For this review, take the finished solid that the model builds, in its own axes (mm). Face numbers are marked on the shaded views. A direction names the side the tool comes from. Give positions to 0.01 mm unless a question says otherwise; leave off trailing zeros. Write each loop counter-clockwise with the first axis right and the second up, starting at its lowest first coordinate (ties: lowest second). Pieces come first, ordered by that corner, then holes.
Q1. Insertion check: P1, Ø3.5, axis at x = -21.5, z = 28.5, coming from the -Y side; P2, Ø6, axis at y = -54.5, z = 14, coming from the -X side; P3, Ø2, axis at y = -6.5, z = -4, coming from the +X side; P4, Ø6.5, axis at y = -50.5, z = 30.5, coming from the -X side. Each pin has a flat end and moves straight along its axis. Give the tip position at first contact, or say it passes through.
Q2. We need section A-A (y = -12.5). Give the number of separate pieces and of enclosed holes in the cut face, then the cut area to 3 significant figures.
Q3. For line 1 (X direction, y = -34.5, z = 25.5); line 2 (X direction, y = -20, z = 0) (3 decimals); line 3 (Y direction, x = 6, z = -21) (3 decimals), list the stretches that pass through material, from the lowest coordinate up.
Q4. Mouldability with a two-part tool opening along Y and no side actions: class the marked faces 5, 6 and 7 as released by +Y, released by -Y, zero draft, split by the parting line, or undercut.
Q5. We need section C-C (y = -2). Write out the cut boundary in (x, z), then the cut area to 3 significant figures.
Q6. Machinability: for the marked faces 1, 2, 3 and 4, which of the approach directions +Z, -Z, +X, -X, +Y, -Y give a long, thin tool a straight path to every point of the face, cutting with its end or side? Answer none if there is none.
```python
from build123d import *

# Parameters (mm, degrees)
BASE_EXTRUDE_DEPTH              = 33.02
SKETCH3_OUTSIDE_W               = 90.796
SKETCH3_OUTSIDE_H               = 92.225
CUT_EXTRUDE1_DEPTH              = 84.020179032
FILLET1_R                       = 3.175
SHELL1_START                    = -64
SHELL1_DEPTH                    = 60.825
CUT_EXTRUDE2_DEPTH              = 90.002703004
BOSS_EXTRUDE2_REACH             = 82.294
SKETCH5_R                       = 4.7625
BOSS_EXTRUDE2_DIRECTION_2_REACH = 82.294
BOSS_EXTRUDE3_DEPTH             = 3.175
SKETCH7_R                       = 6.35
BOSS_EXTRUDE4_DEPTH             = 4.7625


with BuildPart() as part:
    # Sketch2 → Base-Extrude (new, symmetric)
    with BuildSketch(Plane.ZY):
        with BuildLine():
            Line((-25.4, 0), (31.75, 0))
            Line((31.75, 0), (41.801384237, -48.20777973))
            ThreePointArc((41.801384237, -48.20777973), (33.708556891, -62.735496477), (18.174681196, -56.798568464))
            ThreePointArc((18.174681196, -56.798568464), (-0.820496403, -29.162568375), (-25.4, -6.35))
            Line((-25.4, -6.35), (-25.4, 0))
        make_face()
    extrude(amount=BASE_EXTRUDE_DEPTH, both=True)

    # Sketch3 outside → Cut-Extrude1 (cut, through all)
    with BuildSketch(Plane(origin=(0, 0, 0), x_dir=(-1, 0, 0), z_dir=(0, 1, 0))):
        with Locations((0, 8.3345)):
            Rectangle(SKETCH3_OUTSIDE_W, SKETCH3_OUTSIDE_H)
        with BuildLine():
            Line((20.6375, 14.807214247), (20.6375, 48.151384237))
            Line((20.6375, 48.151384237), (-20.6375, 48.151384237))
            Line((-20.6375, 48.151384237), (-20.6375, 14.807214247))
            ThreePointArc((-20.6375, 14.807214247), (0, -25.4), (20.6375, 14.807214247))
        make_face(mode=Mode.SUBTRACT)
    extrude(amount=-CUT_EXTRUDE1_DEPTH, mode=Mode.SUBTRACT)

    # Fillet1
    # the kernel refuses this fillet: 3.175 mm, written as the material it adds along each edge
    with BuildSketch(Plane(origin=(20.6375, 0, 14.807214247), x_dir=(0.567961525786319, 0, -0.8230551046111534), z_dir=(0, -1, 0))) as fillet1_piece_1_section:
        with BuildLine():
            CenterArc((0.989925475, 3.174465965), FILLET1_R, 235.391801271, 33.557309762)
            Line((-0.813352369, 0.561266008), (0, 0))
            ThreePointArc((0, 0), (0.465847282, 0.004272282), (0.931694565, 0))
        make_face()
    fillet1_piece_1 = extrude(amount=53.310385567, mode=Mode.PRIVATE)
    fillet1_piece_1 = fillet1_piece_1 - Plane(origin=(20.6375, -128.781390034, -116.154144448), x_dir=(0, 0.4723282255219985, 0.8814227404459453), z_dir=(-1, 0, 0)) * Cylinder(152.4, 111, mode=Mode.PRIVATE)
    add(fillet1_piece_1)
    with BuildSketch(Plane(origin=(-20.6375, 0, 14.807214247), x_dir=(-0.5679615257863165, 0, -0.8230551046111549), z_dir=(0, -1, 0))) as fillet1_piece_2_section:
        with BuildLine():
            CenterArc((0.989925475, -3.174465965), FILLET1_R, 91.050888967, 33.557309762)
            Line((-0.813352369, -0.561266008), (0, 0))
            ThreePointArc((0, 0), (0.465847282, -0.004272282), (0.931694565, 0))
        make_face()
    fillet1_piece_2 = extrude(amount=53.310385567, mode=Mode.PRIVATE)
    fillet1_piece_2 = fillet1_piece_2 - Plane(origin=(-20.6375, -128.781390034, -116.154144448), x_dir=(0, 0.4723282255219985, 0.8814227404459453), z_dir=(-1, 0, 0)) * Cylinder(152.4, 111, mode=Mode.PRIVATE)
    add(fillet1_piece_2)
    # the kernel refuses this fillet: 3.175 mm, written as the material it takes off along each edge
    with BuildSketch(Plane(origin=(0, 0, 0), x_dir=(-0.8333333333333335, 0, 0.5527707983925666), z_dir=(0.5527707983925666, 0, 0.8333333333333335))) as fillet1_2_piece_1:
        with BuildLine():
            CenterArc((25.4 - FILLET1_R, FILLET1_R), FILLET1_R, 270, 90)
            Line((25.4 - FILLET1_R, 0), (25.4, 0))
            Line((25.4, 0), (25.4, FILLET1_R))
        make_face()
    revolve(axis=Axis((0, 0, 0), (0, -1, 0)), revolution_arc=247.114619524, mode=Mode.SUBTRACT)
    with BuildSketch(Plane(origin=(20.6375, 0, 39.6875), x_dir=(-1, 0, 0), z_dir=(0, 0, -1)), Plane(origin=(-20.6375, 0, 15.795425564), x_dir=(1, 0, 0), z_dir=(0, 0, 1))) as fillet1_2_piece_2:
        with BuildLine():
            CenterArc((FILLET1_R, -FILLET1_R), FILLET1_R, 90, 90)
            Line((0, -FILLET1_R), (0, 0))
            Line((0, 0), (FILLET1_R, 0))
        make_face()
    extrude(amount=23.892074436, mode=Mode.SUBTRACT)
    with BuildSketch(Plane(origin=(-23.8125, 0, 15.795425564), x_dir=(0.8333333333333333, 0, -0.5527707983925668), z_dir=(-0.5527707983925668, 0, -0.8333333333333333))) as fillet1_2_piece_3:
        with BuildLine():
            CenterArc((3.175 + FILLET1_R, FILLET1_R), FILLET1_R, 180, 90)
            Line((3.175, FILLET1_R), (3.175, 0))
            Line((3.175, 0), (3.175 + FILLET1_R, 0))
        make_face()
    revolve(axis=Axis((-23.8125, 0, 15.795425564), (0, -1, 0)), revolution_arc=33.557309762, mode=Mode.SUBTRACT)
    with BuildSketch(Plane(origin=(23.8125, 0, 15.795425564), x_dir=(-0.8333333333333333, 0, -0.5527707983925668), z_dir=(0.5527707983925668, 0, -0.8333333333333333))) as fillet1_2_piece_4:
        with BuildLine():
            CenterArc((3.175 + FILLET1_R, -FILLET1_R), FILLET1_R, 90, 90)
            Line((3.175, -FILLET1_R), (3.175, 0))
            Line((3.175, 0), (3.175 + FILLET1_R, 0))
        make_face()
    revolve(axis=Axis((23.8125, 0, 15.795425564), (0, 1, 0)), revolution_arc=33.557309762, mode=Mode.SUBTRACT)

    # Shell1: read off the stored shape, not the designer's step
    # Shell1 outline → Shell1 (cut)
    with BuildSketch(Plane(origin=(0, 0, 0), x_dir=(1, 0, 0), z_dir=(0, 1, 0)).offset(SHELL1_START)):
        with BuildLine():
            ThreePointArc((17.4625, -15.795425564), (17.732837866, -13.962338459), (18.520833333, -12.285330994))
            ThreePointArc((18.520833333, -12.285330994), (0, 22.225), (-18.520833333, -12.285330994))
            ThreePointArc((-18.520833333, -12.285330994), (-17.732837866, -13.962338459), (-17.4625, -15.795425564))
            Line((-17.4625, -15.795425564), (-17.4625, -44))
            Line((-17.4625, -44), (17.4625, -44))
            Line((17.4625, -44), (17.4625, -15.795425564))
        make_face()
    extrude(amount=SHELL1_DEPTH, mode=Mode.SUBTRACT)

    # Sketch4 → Cut-Extrude2 (cut, through all)
    with BuildSketch(Plane.ZY.offset(-20.6375)):
        with BuildLine():
            Line((24.14125847, -10.173055068), (28.029588875, -28.822006423))
            ThreePointArc((28.029588875, -28.822006423), (31.785802502, -31.282109915), (34.245905994, -27.525896288))
            Line((34.245905994, -27.525896288), (30.357575589, -8.876944932))
            ThreePointArc((30.357575589, -8.876944932), (26.601361962, -6.416841441), (24.14125847, -10.173055068))
        make_face()
    extrude(amount=CUT_EXTRUDE2_DEPTH, mode=Mode.SUBTRACT)

    # Sketch5 → Boss-Extrude2 (add, up to next)
    with BuildSketch(Plane(origin=(0, 0, 0), x_dir=(0, 0, -1), z_dir=(1, 0, 0)), mode=Mode.PRIVATE) as boss_extrude2_sk1:
        with Locations((-29.36875, -50.8)):
            Circle(SKETCH5_R)
    boss_extrude2_tool1 = extrude(boss_extrude2_sk1.sketch, amount=BOSS_EXTRUDE2_REACH, mode=Mode.PRIVATE) - part.part
    add(boss_extrude2_tool1.solids().sort_by_distance((0, -50.8, 29.36875))[0])

    # Sketch5 → Boss-Extrude2 direction 2 (add, up to next)
    with BuildSketch(Plane(origin=(0, 0, 0), x_dir=(0, 0, -1), z_dir=(1, 0, 0)), mode=Mode.PRIVATE) as boss_extrude2_direction_2_sk1:
        with Locations((-29.36875, -50.8)):
            Circle(SKETCH5_R)
    boss_extrude2_direction_2_tool1 = extrude(boss_extrude2_direction_2_sk1.sketch, amount=-BOSS_EXTRUDE2_DIRECTION_2_REACH, mode=Mode.PRIVATE) - part.part
    add(boss_extrude2_direction_2_tool1.solids().sort_by_distance((0, -50.8, 29.36875))[0])

    # Sketch6 → Boss-Extrude3 (add)
    with BuildSketch(Plane.ZY.offset(20.6375)):
        Polygon((33.034924209, -44.45), (25.702575791, -44.45), (22.036401581, -50.8), (25.702575791, -57.15), (33.034924209, -57.15), (36.701098419, -50.8), align=None)
    boss_extrude3 = extrude(amount=BOSS_EXTRUDE3_DEPTH)

    # Mirror1: Boss-Extrude3 across plane
    add(boss_extrude3.mirror(Plane(origin=(0, 0, 0), x_dir=(0, 0, 1), z_dir=(1, 0, 0))))

    # Sketch7 → Boss-Extrude4 (add)
    with BuildSketch(Plane(origin=(0, 0, 0), x_dir=(-1, 0, 0), z_dir=(0, 1, 0))):
        with Locations(Location((0, 0, 0), (0, 0, 270))):
            Circle(SKETCH7_R)
    extrude(amount=BOSS_EXTRUDE4_DEPTH)


solid = part.part
```
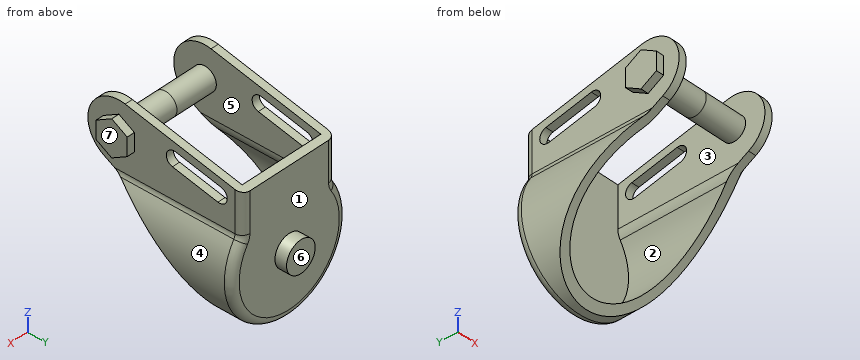
Computed:
1. P1: stops at y = -63.5
1. P2: stops at x = -20.66
1. P3: stops at x = 25.22
1. P4: stops at x = -23.81
2. separate pieces: 4
2. enclosed holes: 0
2. area: 309 mm2
3. line 1: x = -20.64 to -17.46, 17.46 to 20.64
3. line 2: x = -25.4 to -22.225, 22.225 to 25.4
3. line 3: y = -3.175 to 0
4. face 5: undercut
4. face 6: released by +Y
4. face 7: zero draft
5. outline: (-20.98, 13.92) arc R25.17 ccw (long way) to (20.98, 13.92) arc R3.4 cw to (20.41, 15.8) - (20.41, 32.17) - (-20.41, 32.17) - (-20.41, 15.8) arc R3.4 cw to start
5. area: 2,400 mm2
6. face 1: +Y
6. face 2: -Y
6. face 3: none
6. face 4: +Y, -Y
